Read the model definition and answer for the solid it produces. Units are mm, in the model's axes. A direction names the side the tool comes from. Coordinates: 2 decimals unless noted, no trailing zeros. Loops run counter-clockwise (first coordinate to the right, second up) from the corner with the lowest first, then second, coordinate; pieces in that order, holes last. Notation, with made-up numbers: M 81.5,39.5 L 109.5,39.5 A20 cw 109.5,51.5 Z; hole C -12.75,49.25 d9. An arc over 180 degrees is marked long. Use one line per item in the form item = value. Start each with the question number.
1. Flat-ended cylindrical pins translate along their axes: pin 1 (9 mm diameter, centred on y = -10, z = -90.5, fed in from -X); pin 2 (9 mm diameter, centred on x = -46, y = -21.5, fed in from +Z); pin 3 (12 mm diameter, centred on y = -10, z = -63, fed in from -X). Find the tip coordinate at first contact, or state that the pin passes through.
2. The part is cut by section B-B (z = -74). Give the vertices of the cut face in (x, y), plus the area to 3 significant figures.
3. A tool of negligible diameter and unlimited length cuts with its end or side. For faces 1 (the flat face through (-55, -15, 48.034)), 2 (the flat face through (149.42, -15, -87)), 3 (the flat face through (-90.58, -15, -87)), 4 (the cylindrical face through (95.64, -14.79, -95.25)), 5 (the cylindrical face through (-112.27, -14.79, -31.41)), from which of +Z, -Z, +X, -X, +Y, -Y can it reach the whole face along a straight path? Write none if from no direction.
4. The part is cut by section C-C (y = -15.5). Give the number of separate pieces and of enclosed holes in the cut face, plus the area to 3 significant figures.
5. Find the intervals of material crossed by probe 1 along X at (y, z) = (-19.5, -62.5); probe 2 along X at (y, z) = (-4.75, -44.5); probe 3 along X at (y, z) = (-4, -55), in increasing order. Write a range as [from, to].
6. For a pull along Z with two mould halves and no side action, classify faces 6 (the flat face through (-56, -15, -111.966)), 7 (the flat face through (-5, 0, -30)), 8 (the flat face through (-56, -15, 33.034)) as released by +Z, released by -Z, zero draft, split by the parting line, or undercut.
7. The part is cut by section A-A (x = 125). Give the vertices of the cut face in (y, z).
8. The part is cut by section D-D (z = 44). Give the vertices of the cut face in (x, y).
from build123d import *

# Parameters (mm, degrees)
F0_R     = 30
F1_DEPTH = 30


with BuildPart() as f1:
    # F0 (on Front) → F1 (new body)
    with BuildSketch(Plane.XZ):
        with BuildLine():
            ThreePointArc((79.419856, 48.034481), (29.419856, 63.916465), (-20.580144, 48.034481))
            Line((-20.580144, 48.034481), (-90.580144, 48.034481))
            Line((-90.580144, 48.034481), (-90.580144, -1.965519))
            ThreePointArc((-90.580144, -1.965519), (-112.275858, -31.965519), (-90.580144, -61.965519))
            Line((-90.580144, -61.965519), (-90.580144, -111.965519))
            Line((-90.580144, -111.965519), (-20.580144, -111.965519))
            ThreePointArc((-20.580144, -111.965519), (29.419856, -126.504106), (79.419856, -111.965519))
            Line((79.419856, -111.965519), (149.419856, -111.965519))
            Line((149.419856, -111.965519), (149.419856, -61.965519))
            ThreePointArc((149.419856, -61.965519), (169.267812, -31.965519), (149.419856, -1.965519))
            Line((149.419856, -1.965519), (149.419856, 48.034481))
            Line((149.419856, 48.034481), (79.419856, 48.034481))
        make_face()
        with BuildLine():
            ThreePointArc((-75.580144, 27.034481), (-73.822784, 31.277122), (-69.580144, 33.034481))
            Line((-69.580144, 33.034481), (-43.045036, 33.034481))
            ThreePointArc((-43.045036, 33.034481), (-38.802395, 31.277122), (-37.045036, 27.034481))
            Line((-37.045036, 27.034481), (-37.045036, -90.965519))
            ThreePointArc((-37.045036, -90.965519), (-38.802395, -95.20816), (-43.045036, -96.965519))
            Line((-43.045036, -96.965519), (-69.580144, -96.965519))
            ThreePointArc((-69.580144, -96.965519), (-73.822784, -95.20816), (-75.580144, -90.965519))
            Line((-75.580144, -90.965519), (-75.580144, 27.034481))
        make_face(mode=Mode.SUBTRACT)
        with Locations((29.419856, -31.965519)):
            Circle(F0_R, mode=Mode.SUBTRACT)
        with BuildLine():
            ThreePointArc((93.84039, 27.034481), (95.59775, 31.277122), (99.84039, 33.034481))
            Line((99.84039, 33.034481), (128.419856, 33.034481))
            ThreePointArc((128.419856, 33.034481), (132.662497, 31.277122), (134.419856, 27.034481))
            Line((134.419856, 27.034481), (134.419856, -90.965519))
            ThreePointArc((134.419856, -90.965519), (132.662497, -95.20816), (128.419856, -96.965519))
            Line((128.419856, -96.965519), (99.84039, -96.965519))
            ThreePointArc((99.84039, -96.965519), (95.59775, -95.20816), (93.84039, -90.965519))
            Line((93.84039, -90.965519), (93.84039, 27.034481))
        make_face(mode=Mode.SUBTRACT)
    extrude(amount=F1_DEPTH)


solid = f1.part
Computed values:
q1.pin_1 = -90.58
q1.pin_2 = 48.03
q1.pin_3 = -99.95
q2.outline = M -90.58,-30 L -75.58,-30 L -75.58,0 L -90.58,0 Z; M -37.05,-30 L 93.84,-30 L 93.84,0 L -37.05,0 Z; M 134.42,-30 L 149.42,-30 L 149.42,0 L 134.42,0 Z
q2.area = 4,830 mm²
q3.face_1 = +Z, -X, +Y, -Y
q3.face_2 = -Z, +X, +Y, -Y
q3.face_3 = -Z, -X, +Y, -Y
q3.face_4 = +Y, -Y
q3.face_5 = -X, +Y, -Y
q4.separate_pieces = 1
q4.enclosed_holes = 3
q4.area = 29,200 mm²
q5.probe_1 = [-90.58, -75.58], [-37.05, 93.84], [134.42, 149.42]
q5.probe_2 = [-109.68, -75.58], [-37.05, 2.16], [56.68, 93.84], [134.42, 166.76]
q5.probe_3 = [-102.3, -75.58], [-37.05, 10.2], [48.64, 93.84], [134.42, 159.74]
q6.face_6 = released by -Z
q6.face_7 = zero draft
q6.face_8 = undercut
q7.outline = M -30,-111.97 L 0,-111.97 L 0,-96.97 L -30,-96.97 Z; M -30,33.03 L 0,33.03 L 0,48.03 L -30,48.03 Z
q8.outline = M -90.58,-30 L 149.42,-30 L 149.42,0 L -90.58,0 Z
